CAD build for the part. Positions are in the model's coordinates, mm. Face numbers are marked on the shaded views. A direction names the side the tool comes from. Round coordinates to 2 decimals unless told otherwise and drop trailing zeros. Order: outer loops, then holes, each group sorted by start corner. A loop starts at its lowest first (then second) coordinate and runs counter-clockwise, first axis right, second up. Notation, with made-up numbers: M 38,89 L 57,89 A19 cw 57,113 Z; hole C -19,-0.75 d3. An arc over 180 degrees is marked long. Put each result on its own line as item: value.
```python
from build123d import *

# Parameters (mm, degrees)
SKETCH1_R               = 8
BOSS_EXTRUDE1_DEPTH     = 82
SKETCH2_R               = 6
BOSS_EXTRUDE2_DEPTH     = 10
SKETCH4_R               = 9
BOSS_EXTRUDE3_DEPTH     = 24
SKETCH5_R               = 6
BOSS_EXTRUDE4_DEPTH     = 10
SKETCH6_R               = 4
BOSS_EXTRUDE5_DEPTH     = 6
SKETCH7_R               = 6
BOSS_EXTRUDE6_DEPTH     = 7
SKETCH8_R               = 3
CUT_EXTRUDE2_DEPTH      = 10
CUT_EXTRUDE2_DEPTH_BACK = 10


with BuildPart() as part:
    # Sketch1 → Boss-Extrude1 (new body)
    with BuildSketch(Plane(origin=(0, 0, 0), x_dir=(1, 0, 0), z_dir=(0, 1, 0))):
        Circle(SKETCH1_R)
    extrude(amount=BOSS_EXTRUDE1_DEPTH)

    # Sketch2 → Boss-Extrude2 (add)
    with BuildSketch(Plane(origin=(0, 82, 0), x_dir=(1, 0, 0), z_dir=(0, 1, 0))):
        Circle(SKETCH2_R)
    extrude(amount=BOSS_EXTRUDE2_DEPTH)

    # Sketch4 → Boss-Extrude3 (add)
    with BuildSketch(Plane(origin=(0, 92, 0), x_dir=(1, 0, 0), z_dir=(0, 1, 0))):
        Circle(SKETCH4_R)
    extrude(amount=BOSS_EXTRUDE3_DEPTH)

    # Sketch5 → Boss-Extrude4 (add)
    with BuildSketch(Plane.XZ):
        Circle(SKETCH5_R)
    extrude(amount=BOSS_EXTRUDE4_DEPTH)

    # Sketch6 → Boss-Extrude5 (add)
    with BuildSketch(Plane.XZ.offset(10)):
        Circle(SKETCH6_R)
    extrude(amount=BOSS_EXTRUDE5_DEPTH)

    # Sketch7 → Boss-Extrude6 (add)
    with BuildSketch(Plane.XZ.offset(16)):
        Circle(SKETCH7_R)
    extrude(amount=BOSS_EXTRUDE6_DEPTH)

    # Sketch8 → Cut-Extrude2 (cut, two sides)
    with BuildSketch(Plane.XY) as cut_extrude2_sk:
        with Locations((0, 104)):
            Circle(SKETCH8_R)
    extrude(amount=CUT_EXTRUDE2_DEPTH, mode=Mode.SUBTRACT)
    extrude(cut_extrude2_sk.sketch, amount=-CUT_EXTRUDE2_DEPTH_BACK, mode=Mode.SUBTRACT)


solid = part.part
```
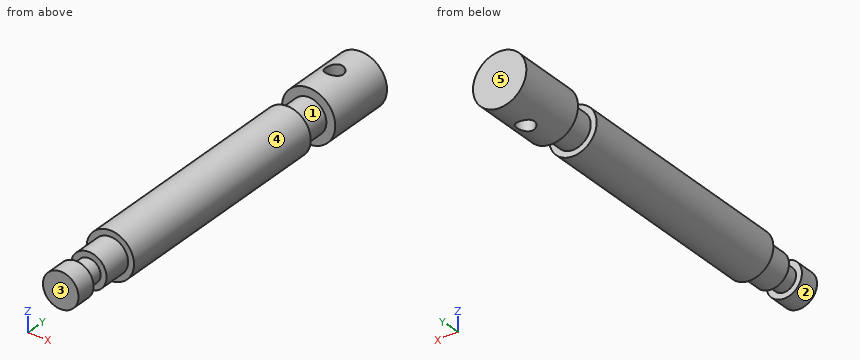
Item 1: Tool access for the marked faces 4 and 5: list every direction of +Z, -Z, +X, -X, +Y, -Y with a clear straight run to the whole face (end or side of a thin tool).
Answers below:
face 4: -Y
face 5: +Z, -Z, +X, -X, +Y
Item 2: Mould opens along Y. For the marked faces 1, 2 and 3 say: pulls with the +Y half, pulls with the -Y half, needs draft (parallel to the pull), parting line crosses it, or undercut.
Answers below:
face 1: undercut
face 2: needs draft
face 3: pulls with the -Y half
Item 3: Band-saw the part on B-B on y = 84. Give the cut face in (x, z), and give its area (3 significant figures).
Answers below:
outline: C 0,0 d12
area: 113 mm²
Item 4: Pin check, flat tips, straight feed: P1, Ø1.5, axis at y = 85, z = -5.5, coming from the -X side; P2, Ø6, axis at y = 83.5, z = -1.5, coming from the -X side; P3, Ø4, axis at y = 88, z = 6.5, coming from the +X side. Stop position of each tip, or through.
Answers below:
P1: x = -3.67
P2: x = -8
P3: x = 3.97
Item 5: Band-saw the part on D-D on y = 8.5. Give the cut face in (x, z), and give its area (3 significant figures).
Answers below:
outline: C 0,0 d16
area: 201 mm²
Item 6: Band-saw the part on A-A on x = 0. Give the cut face in (y, z).
Answers below:
outline: M -23,-6 L -16,-6 L -16,-4 L -10,-4 L -10,-6 L 0,-6 L 0,-8 L 82,-8 L 82,-6 L 92,-6 L 92,-9 L 101,-9 L 101,9 L 92,9 L 92,6 L 82,6 L 82,8 L 0,8 L 0,6 L -10,6 L -10,4 L -16,4 L -16,6 L -23,6 Z; M 107,-9 L 116,-9 L 116,9 L 107,9 Z
Item 7: Probe line 1 along Y through (x, z) = (0, 5.5); line 2 along Y through (x, z) = (0, 7); line 3 along Y through (x, z) = (0, 3.75). List the from-to ranges inside material, lowest first. Write a range as [from, to].
Answers below:
line 1: [-23, -16], [-10, 101], [107, 116]
line 2: [0, 82], [92, 101], [107, 116]
line 3: [-23, 101], [107, 116]
Item 8: Band-saw the part on C-C on y = 104. Give the cut face in (x, z).
Answers below:
outline: M -3,-8.49 L -3,8.49 A9 ccw Z; M 3,-8.49 A9 ccw 3,8.49 Z
